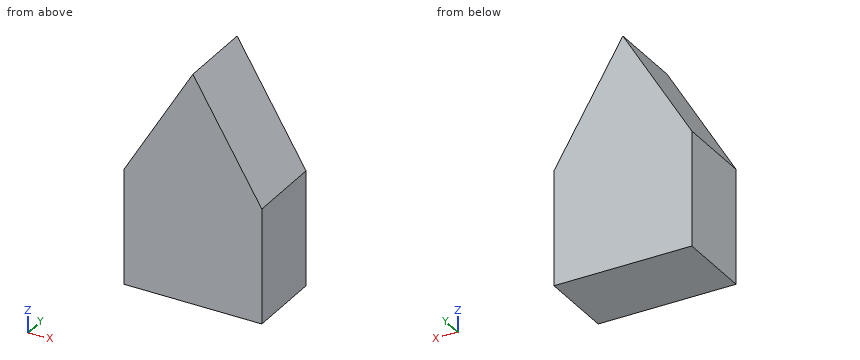
from build123d import *

# Parameters (mm, degrees)
F0_W     = 18
F0_H     = 15
F1_DEPTH = 10


with BuildPart() as f1:
    # F0 (on Front) → F1 (new body)
    with BuildSketch(Plane.XZ):
        Rectangle(F0_W, F0_H)
        Polygon((-9, 7.5), (9, 7.5), (0, 22.5), align=None)
    extrude(amount=F1_DEPTH)


solid = f1.part
Source: CAD feature listing. Evaluate the final solid. Frame: model axes, mm. Give positions to 0.01 mm unless a question says otherwise; leave off trailing zeros. Write each loop counter-clockwise with the first axis right and the second up, starting at its lowest first coordinate (ties: lowest second). Pieces come first, ordered by that corner, then holes. Notation, with made-up numbers: M -38,66 L -15,66 A26 cw -15,85 Z; hole C -30.5,47.25 d4. An arc over 180 degrees is marked long. Return JSON: item names as keys, results as strings. Group by question number.
1) Ray query, L1, parallel to X at y = -7.5, z = 13.5; L2, parallel to Z at x = 5, y = -7.5; L3, parallel to Z at x = 6, y = -2. Return the intervals inside material, ascending.
2) Cut plane C-C, the plane x = 3. Output: boundary loops of the cut face in (y, z), then the cut area to 3 significant figures.
3) First-contact query: pin 1 Ø2 at (y, z) = (-7, 14) entering from -X; pin 2 Ø4 at (y, z) = (-2.5, 13.5) entering from +X. Flat tips, straight axial feed; report the tip coordinate or a pass-through.
4) Cut plane A-A, the plane y = -3.75. Output: boundary loops of the cut face in (x, z).
5) Cut plane B-B, the plane z = 15.5. Output: boundary loops of the cut face in (x, y), then the cut area to 3 significant figures.
Data:
{
 "1": {"L1": "x = -5.4 to 5.4", "L2": "z = -7.5 to 14.17", "L3": "z = -7.5 to 12.5"},
 "2": {"outline": "M -10,-7.5 L 0,-7.5 L 0,17.5 L -10,17.5 Z", "area": "250 mm²"},
 "3": {"pin 1": "stops at x = -5.7", "pin 2": "stops at x = 6.6"},
 "4": {"outline": "M -9,-7.5 L 9,-7.5 L 9,7.5 L 0,22.5 L -9,7.5 Z"},
 "5": {"outline": "M -4.2,-10 L 4.2,-10 L 4.2,0 L -4.2,0 Z", "area": "84.0 mm²"}
}
